Print and shaded views of the part. All mm, measured from the part's lowest x, y and z. A direction names the side the tool comes from. Give positions to 0.01 mm unless a question says otherwise; leave off trailing zeros. Loops run counter-clockwise (first coordinate to the right, second up) from the corner with the lowest first, then second, coordinate; pieces in that order, holes last. Notation, with made-up numbers: (5, -7) -> (59, -7) arc R6 ccw to (59, 4) -> close; hole circle Ø7 at (-29, 50). An arc over 180 degrees is marked (long way). Answer as a JSON object with one key per item and string values. Group by question number.
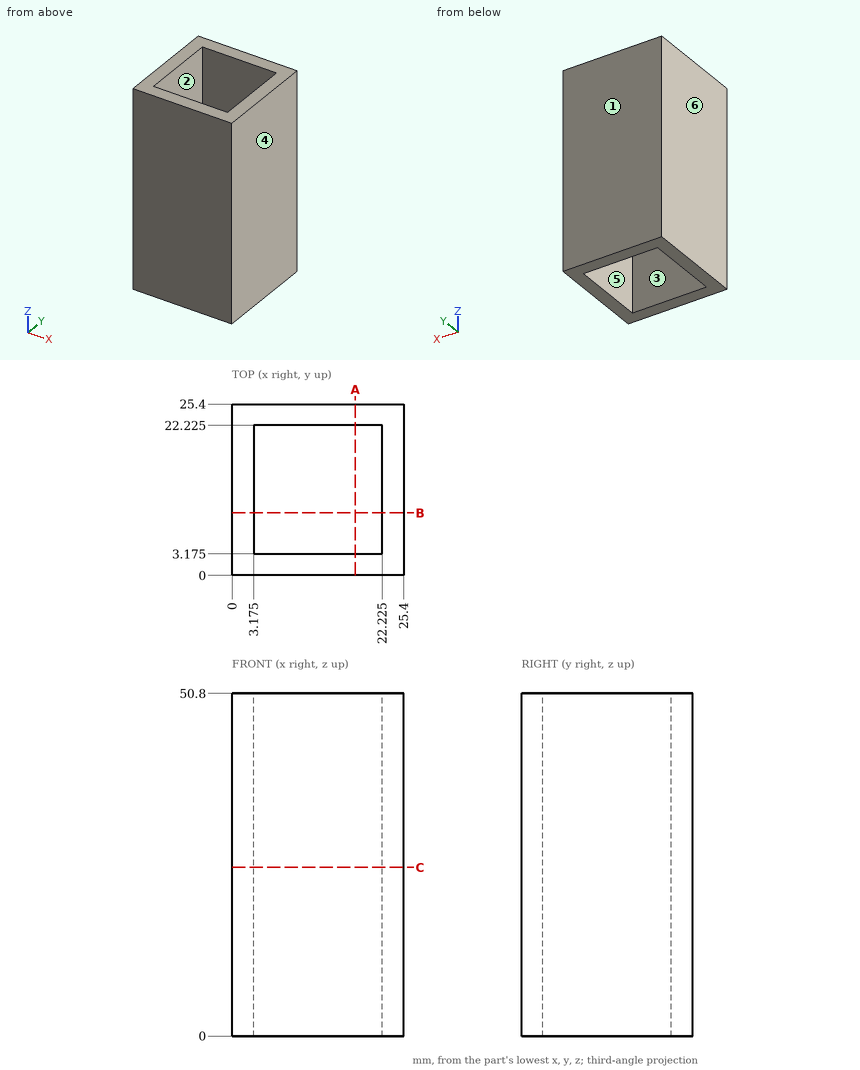
(1) Saw through at C-C on z = 25. List the corners of the cut face in (x, y) (3 decimals).
(2) Probe line 1 along Y through (x, z) = (12.5, 18) (3 decimals). List the from-to ranges inside material, lowest first. Write a range as [from, to].
(3) Pull direction X, two halves, no side cores. Call the marked faces 3, 4, 5 and 6: pulls with the +X half, pulls with the -X half, needs draft (parallel to the pull), parting line crosses it, or undercut.
(4) 3-axis set-ups, long thin cutter, end or side, ignore diameter. For the marked faces 1 and 2: which of +Z, -Z, +X, -X, +Y, -Y reach the whole face in a straight line?
(5) Saw through at A-A on x = 18.25. List the corners of the cut face in (y, z) (3 decimals), plus the area to 3 significant figures.
Calculated:
{
 "1": {"outline": "(0, 0) -> (25.4, 0) -> (25.4, 25.4) -> (0, 25.4) -> close; hole (3.175, 3.175) -> (22.225, 3.175) -> (22.225, 22.225) -> (3.175, 22.225) -> close"},
 "2": {"line 1": "y = [0, 3.175], [22.225, 25.4]"},
 "3": {"face 3": "undercut", "face 4": "pulls with the +X half", "face 5": "undercut", "face 6": "pulls with the -X half"},
 "4": {"face 1": "+Z, -Z, +X, -X, +Y", "face 2": "+Z, -Z"},
 "5": {"outline": "(0, 0) -> (3.175, 0) -> (3.175, 50.8) -> (0, 50.8) -> close; (22.225, 0) -> (25.4, 0) -> (25.4, 50.8) -> (22.225, 50.8) -> close", "area": "323 mm^2"}
}
